from build123d import *

# Parameters (mm, degrees)
BOSS_EXTRUDE1_DEPTH     = 15
CUT_EXTRUDE1_DEPTH      = 1
CUT_EXTRUDE1_DEPTH_BACK = 16


with BuildPart() as part:
    # Sketch1 → Boss-Extrude1 (new body)
    with BuildSketch(Plane.XY):
        with BuildLine():
            Line((-236.729376996, 0), (0, 0))
            Line((0, 0), (357.876847169, 0))
            Line((357.876847169, 0), (396.730398779, 416))
            Line((396.730398779, 416), (315.832809595, 416))
            Line((315.832809595, 416), (236.983089551, 242.144494596))
            ThreePointArc((236.983089551, 242.144494596), (164.696190822, 146.877858304), (58.352308735, 92.177707838))
            Line((58.352308735, 92.177707838), (-236.729376996, 16.274880501))
            Line((-236.729376996, 16.274880501), (-236.729376996, 0))
        make_face()
    extrude(amount=BOSS_EXTRUDE1_DEPTH)

    # Sketch2 → Cut-Extrude1 (cut, two sides)
    with BuildSketch(Plane.XY.offset(15)) as cut_extrude1_sk:
        Polygon((396.730398779, 416), (357.876847169, 0), (296.597151769, 0), (371.734942748, 416), align=None)
    extrude(amount=CUT_EXTRUDE1_DEPTH, mode=Mode.SUBTRACT)
    extrude(cut_extrude1_sk.sketch, amount=-CUT_EXTRUDE1_DEPTH_BACK, mode=Mode.SUBTRACT)


solid = part.part
Part model, mm, in its own coordinate system. Round coordinates to 2 decimals unless told otherwise and drop trailing zeros. Loops run counter-clockwise (first coordinate to the right, second up) from the corner with the lowest first, then second, coordinate; pieces in that order, holes last. Notation, with made-up numbers: (-23.5, 13.25) - (3.5, 13.25) arc R29 ccw to (3.5, 49.25) - close; hole circle Ø9 at (3, -27). An arc over 180 degrees is marked (long way). Answer as a JSON object with one key per item and string values.
Item 1: Band-saw the part on A-A on z = 6. List the corners of the cut face in (x, y).
Output:
{"outline": "(-236.73, 0) - (296.6, 0) - (371.73, 416) - (315.83, 416) - (236.98, 242.14) arc R270 cw to (58.35, 92.18) - (-236.73, 16.27) - close"}
Item 2: Wall check: L1, parallel to X at y = 157.5, z = 3; L2, parallel to X at y = 191, z = 9; L3, parallel to Y at x = -190, z = 4.5. Give the ranges that are in metal, low to high.
Output:
{"L1": "176.61 to 325.04", "L2": "206.59 to 331.1", "L3": "0 to 28.29"}
Item 3: Band-saw the part on B-B on x = -78.5. List the corners of the cut face in (y, z), plus the area to 3 significant figures.
Output:
{"outline": "(0, 0) - (56.98, 0) - (56.98, 15) - (0, 15) - close", "area": "855 mm2"}
Item 4: Band-saw the part on C-C on y = 213.5. List the corners of the cut face in (x, z).
Output:
{"outline": "(221.86, 0) - (335.16, 0) - (335.16, 15) - (221.86, 15) - close"}
Item 5: Pin check, flat tips, straight feed: pin 1 (5 mm diameter, centred on x = -149.5, z = 2, fed in from +Y); pin 2 (3 mm diameter, centred on y = 169.5, z = 3.5, fed in from +X); pin 3 (1 mm diameter, centred on y = 268, z = 11, fed in from -X). Stop position of each tip, or through.
Output:
{"pin 1": "y = 39.36", "pin 2": "x = 327.48", "pin 3": "x = 248.48"}
